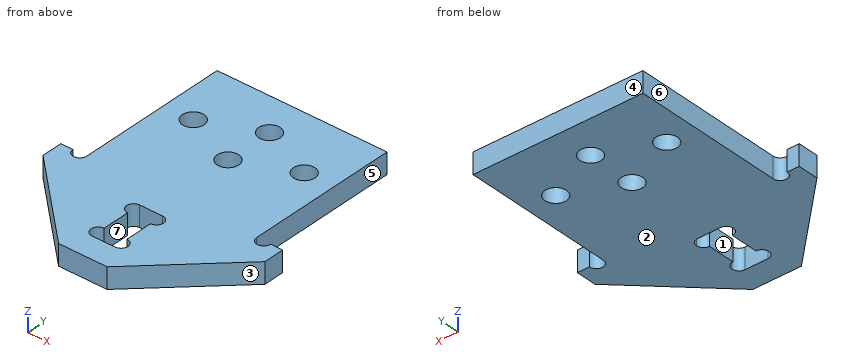
```python
from build123d import *

# Parameters (mm, degrees)
SKETCH_1_R      = 1.55
EXTRUDE_1_DEPTH = 3


with BuildPart() as part:
    # 草图1 → 凸台-拉伸1 (new body)
    with BuildSketch(Plane.XY):
        with BuildLine():
            Line((-12.25, 11), (-12.25, -11))
            ThreePointArc((-12.25, -11), (-13.255, -12.005), (-14.26, -11))
            Line((-14.26, -11), (-16, -11))
            Line((-16, -11), (-16, -14))
            Line((-16, -14), (-3.5, -26))
            Line((-3.5, -26), (3.5, -26))
            Line((3.5, -26), (16, -14))
            Line((16, -14), (16, -11))
            Line((16, -11), (14.26, -11))
            ThreePointArc((14.26, -11), (13.255, -12.005), (12.25, -11))
            Line((12.25, -11), (12.25, 11))
            Line((12.25, 11), (-12.25, 11))
        make_face()
        with BuildLine():
            ThreePointArc((2.655, -21.495), (2.360642315, -22.205642315), (1.65, -22.5))
            Line((1.65, -22.5), (-1.65, -22.5))
            ThreePointArc((-1.65, -22.5), (-2.655, -21.495), (-1.65, -20.49))
            Line((-1.65, -20.49), (-1.65, -16.51))
            ThreePointArc((-1.65, -16.51), (-2.655, -15.505), (-1.65, -14.5))
            Line((-1.65, -14.5), (1.65, -14.5))
            ThreePointArc((1.65, -14.5), (2.360642315, -14.794357685), (2.655, -15.505))
            ThreePointArc((2.655, -15.505), (2.360642315, -16.215642315), (1.65, -16.51))
            Line((1.65, -16.51), (1.65, -20.49))
            ThreePointArc((1.65, -20.49), (2.360642315, -20.784357685), (2.655, -21.495))
        make_face(mode=Mode.SUBTRACT)
        with Locations((-8, 2)):
            Circle(SKETCH_1_R, mode=Mode.SUBTRACT)
        with Locations((0, -1.5)):
            Circle(SKETCH_1_R, mode=Mode.SUBTRACT)
        with Locations((0, 5.5)):
            Circle(SKETCH_1_R, mode=Mode.SUBTRACT)
        with Locations((8, 2)):
            Circle(SKETCH_1_R, mode=Mode.SUBTRACT)
    extrude(amount=EXTRUDE_1_DEPTH)


solid = part.part
```
The listing builds one solid part. Answer for the finished solid, in the listing's coordinates (mm). Face numbers are marked on the shaded views. A direction names the side the tool comes from. Give positions to 0.01 mm unless a question says otherwise; leave off trailing zeros. Write each loop counter-clockwise with the first axis right and the second up, starting at its lowest first coordinate (ties: lowest second). Pieces come first, ordered by that corner, then holes. Notation, with made-up numbers: (57.25, 17.5) -> (80.25, 17.5) arc R27 ccw to (80.25, 44.5) -> close; hole circle Ø2 at (80, -38.75). An arc over 180 degrees is marked (long way). Use one line per item in the form item = value.
1) A tool of negligible diameter and unlimited length cuts with its end or side. For the marked faces 4, 5, 6 and 7, from which of +Z, -Z, +X, -X, +Y, -Y can it reach the whole face along a straight path? Write none if from no direction.
Result:
face_4 = +Z, -Z, +X, -X, +Y
face_5 = +Z, -Z, +X, +Y
face_6 = +Z, -Z, -X, +Y
face_7 = +Z, -Z
2) Section D-D on x = -8.5 is taken. Write down the section's boundary in (y, z), plus the area to 3 significant figures.
Result:
outline = (-21.2, 0) -> (0.53, 0) -> (0.53, 3) -> (-21.2, 3) -> close; (3.47, 0) -> (11, 0) -> (11, 3) -> (3.47, 3) -> close
area = 87.8 mm²
3) Straight lines are drawn through the part: probe 1 along Y at (x, z) = (0, 2.05); probe 2 along Y at (x, z) = (8.5, 0.5); probe 3 along X at (y, z) = (-9, 0.95). For each, find the intervals that lie inside material, in ascending order.
Result:
probe_1 = -26 to -22.5, -14.5 to -3.05, 0.05 to 3.95, 7.05 to 11
probe_2 = -21.2 to 0.53, 3.47 to 11
probe_3 = -12.25 to 12.25
4) Section C-C on z = 1.65 is taken. Write down the section's boundary in (x, y) (3 decimals).
Result:
outline = (-16, -14) -> (-3.5, -26) -> (3.5, -26) -> (16, -14) -> (16, -11) -> (14.26, -11) arc R1.005 cw to (12.25, -11) -> (12.25, 11) -> (-12.25, 11) -> (-12.25, -11) arc R1.005 cw to (-14.26, -11) -> (-16, -11) -> close; hole circle Ø3.1 at (-8, 2); hole (-1.65, -22.5) -> (1.65, -22.5) arc R1.005 ccw to (1.65, -20.49) -> (1.65, -16.51) arc R1.005 ccw to (1.65, -14.5) -> (-1.65, -14.5) arc R1.005 ccw to (-1.65, -16.51) -> (-1.65, -20.49) arc R1.005 ccw to start; hole circle Ø3.1 at (0, -1.5); hole circle Ø3.1 at (0, 5.5); hole circle Ø3.1 at (8, 2)
5) For a pull along Y with two mould halves and no side action, classify the marked faces 1, 2 and 3 as +Y half, -Y half, draft (parallel to the pull), parting line (faces both ways), or undercut.
Result:
face_1 = undercut
face_2 = draft
face_3 = -Y half
6) Each of these flat-tipped pins is pushed along its axis until it touches: P1, Ø1.5, axis at y = -2.5, z = 2, coming from the +X side; P2, Ø1.4, axis at x = 15, z = 2, coming from the +Y side; P3, Ø1.5, axis at y = -18.5, z = 2, coming from the -X side. Where does it stop, or does it pass through?
Result:
P1 = 12.25
P2 = -11
P3 = -12.09
7) Section A-A on y = 2 is taken. Write down the section's boundary in (x, z), plus the area to 3 significant figures.
Result:
outline = (-12.25, 0) -> (-9.55, 0) -> (-9.55, 3) -> (-12.25, 3) -> close; (-6.45, 0) -> (6.45, 0) -> (6.45, 3) -> (-6.45, 3) -> close; (9.55, 0) -> (12.25, 0) -> (12.25, 3) -> (9.55, 3) -> close
area = 54.9 mm²
8) Section B-B on x = 8 is taken. Write down the section's boundary in (y, z).
Result:
outline = (-21.68, 0) -> (0.45, 0) -> (0.45, 3) -> (-21.68, 3) -> close; (3.55, 0) -> (11, 0) -> (11, 3) -> (3.55, 3) -> close
